Build history of the part. All positions in model axes, mm. Face numbers are marked on the shaded views. A direction names the side the tool comes from. Give positions to 0.01 mm unless a question says otherwise; leave off trailing zeros. Order: outer loops, then holes, each group sorted by start corner. A loop starts at its lowest first (then second) coordinate and runs counter-clockwise, first axis right, second up. Notation, with made-up numbers: (18.5, 55) -> (49.5, 55) arc R22 ccw to (49.5, 64) -> close; hole circle Ø11 at (11.5, -38.5). An arc over 180 degrees is marked (long way). One line per item, written item: value. Start each with the question number.
(1) Probe line 1 (Z direction, x = -115.5, y = -19.5); line 2 (Y direction, x = -63, z = 14); line 3 (Y direction, x = -143.5, z = 17.5). List the from-to ranges inside material, lowest first.
(2) Which spindle directions (+Z, -Z, +X, -X, +Y, -Y) get a long thin tool onto all of the face, cutting with end or side? Do the marked faces 1, 2 and 3. Say none if no direction does.
(3) Saw through at D-D on z = 23.5. Give the cut face in (x, y).
(4) Saw through at A-A on x = 24.5. Give the cut face in (y, z), plus the area to 3 significant figures.
(5) Pin check, flat tips, straight feed: pin 1 (1.5 mm diameter, centred on y = -13.5, z = 4, fed in from -X); pin 2 (4 mm diameter, centred on y = 19.5, z = 11, fed in from +X); pin 3 (8 mm diameter, centred on x = 22.5, z = 10, fed in from -Y). Stop position of each tip, or through.
(6) Two-plate mould, pull along Y, no slides. Class the marked faces 4, 5, 6 and 7: +Y half, -Y half, draft (parallel to the pull), parting line (faces both ways), or undercut.
(7) Saw through at C-C on x = -23. Give the cut face in (y, z), plus the area to 3 significant figures.
(8) Saw through at B-B on y = -61. Give the cut face in (x, z), plus the area to 3 significant figures.
```python
from build123d import *

# Parameters (mm, degrees)
BOSS_EXTRUDE1_DEPTH = 30
BOSS_EXTRUDE2_DEPTH = 2


with BuildPart() as part:
    # Sketch1 → Boss-Extrude1 (new body)
    with BuildSketch(Plane.XY):
        with BuildLine():
            ThreePointArc((-124.422839539, -52.93360637), (-124.888175134, -64.31939994), (-119.594822483, -74.410646153))
            Line((-119.594822483, -74.410646153), (-111.407238253, -83.286865316))
            Line((-111.407238253, -83.286865316), (35.730934718, -56.776536745))
            Line((35.730934718, -56.776536745), (37.30735825, -35.897821688))
            ThreePointArc((37.30735825, -35.897821688), (33.813482954, -35.461340503), (30.378958676, -34.685632184))
            Line((30.378958676, -34.685632184), (29.158639343, -50.847976334))
            Line((29.158639343, -50.847976334), (-108.867065108, -75.716483958))
            Line((-108.867065108, -75.716483958), (-114.449508902, -69.664516346))
            ThreePointArc((-114.449508902, -69.664516346), (-118.058612981, -62.784121201), (-117.741338712, -55.021080131))
            ThreePointArc((-117.741338712, -55.021080131), (-120.686835144, -35.887822689), (-137.611023, -26.489452883))
            ThreePointArc((-137.611023, -26.489452883), (-140.360427807, -25.849420576), (-142.716361529, -24.294285714))
            ThreePointArc((-142.716361529, -24.294285714), (-148.157403518, -8.953967174), (-139.001078611, 4.503076521))
            ThreePointArc((-139.001078611, 4.503076521), (-130.143335416, 13.552732011), (-127.741520279, 25.986040624))
            ThreePointArc((-127.741520279, 25.986040624), (-124.12688517, 37.354531527), (-113.359672518, 42.490220779))
            Line((-113.359672518, 42.490220779), (36.615125644, 47.908385572))
            Line((36.615125644, 47.908385572), (35.69634188, 35.73968597))
            ThreePointArc((35.69634188, 35.73968597), (39.20840278, 35.99090031), (42.728206295, 35.897821688))
            Line((42.728206295, 35.897821688), (44.184569482, 55.186414758))
            Line((44.184569482, 55.186414758), (-113.612397826, 49.485657143))
            ThreePointArc((-113.612397826, 49.485657143), (-129.404309715, 41.953312906), (-134.705774542, 25.279526249))
            ThreePointArc((-134.705774542, 25.279526249), (-136.343375771, 16.802270376), (-142.382746132, 10.632050724))
            ThreePointArc((-142.382746132, 10.632050724), (-155.099864059, -8.058287742), (-147.542861296, -29.364285714))
            ThreePointArc((-147.542861296, -29.364285714), (-143.125485566, -32.280163581), (-137.970351553, -33.480224156))
            ThreePointArc((-137.970351553, -33.480224156), (-126.431132561, -39.888203569), (-124.422839539, -52.93360637))
        make_face()
    extrude(amount=BOSS_EXTRUDE1_DEPTH)

    # Sketch4 → Boss-Extrude2 (add)
    with BuildSketch(Plane.XY.offset(30)):
        with BuildLine():
            Line((36.615125644, 47.908385572), (-113.359672518, 42.490220779))
            ThreePointArc((-113.359672518, 42.490220779), (-124.12688517, 37.354531527), (-127.741520279, 25.986040624))
            ThreePointArc((-127.741520279, 25.986040624), (-130.143335416, 13.552732011), (-139.001078611, 4.503076521))
            ThreePointArc((-139.001078611, 4.503076521), (-148.157403518, -8.953967174), (-142.716361529, -24.294285714))
            ThreePointArc((-142.716361529, -24.294285714), (-140.360427807, -25.849420576), (-137.611023, -26.489452883))
            ThreePointArc((-137.611023, -26.489452883), (-120.686835144, -35.887822689), (-117.741338712, -55.021080131))
            ThreePointArc((-117.741338712, -55.021080131), (-118.058612981, -62.784121201), (-114.449508902, -69.664516346))
            Line((-114.449508902, -69.664516346), (-108.867065108, -75.716483958))
            Line((-108.867065108, -75.716483958), (29.158639343, -50.847976334))
            Line((29.158639343, -50.847976334), (30.378958676, -34.685632184))
            ThreePointArc((30.378958676, -34.685632184), (4.119960585, 2.710424022), (35.69634188, 35.73968597))
            Line((35.69634188, 35.73968597), (36.615125644, 47.908385572))
        make_face()
        with BuildLine():
            ThreePointArc((-117.741338712, -55.021080131), (-120.686835144, -35.887822689), (-137.611023, -26.489452883))
            ThreePointArc((-137.611023, -26.489452883), (-140.360427807, -25.849420576), (-142.716361529, -24.294285714))
            ThreePointArc((-142.716361529, -24.294285714), (-148.157403518, -8.953967174), (-139.001078611, 4.503076521))
            ThreePointArc((-139.001078611, 4.503076521), (-130.143335416, 13.552732011), (-127.741520279, 25.986040624))
            ThreePointArc((-127.741520279, 25.986040624), (-124.12688517, 37.354531527), (-113.359672518, 42.490220779))
            Line((-113.359672518, 42.490220779), (36.615125644, 47.908385572))
            Line((36.615125644, 47.908385572), (35.69634188, 35.73968597))
            ThreePointArc((35.69634188, 35.73968597), (39.20840278, 35.99090031), (42.728206295, 35.897821688))
            Line((42.728206295, 35.897821688), (44.184569482, 55.186414758))
            Line((44.184569482, 55.186414758), (-113.612397826, 49.485657143))
            ThreePointArc((-113.612397826, 49.485657143), (-129.404309715, 41.953312906), (-134.705774542, 25.279526249))
            ThreePointArc((-134.705774542, 25.279526249), (-136.343375771, 16.802270376), (-142.382746132, 10.632050724))
            ThreePointArc((-142.382746132, 10.632050724), (-155.099864059, -8.058287742), (-147.542861296, -29.364285714))
            ThreePointArc((-147.542861296, -29.364285714), (-143.125485566, -32.280163581), (-137.970351553, -33.480224156))
            ThreePointArc((-137.970351553, -33.480224156), (-126.431132561, -39.888203569), (-124.422839539, -52.93360637))
            ThreePointArc((-124.422839539, -52.93360637), (-124.888175134, -64.31939994), (-119.594822483, -74.410646153))
            Line((-119.594822483, -74.410646153), (-111.407238253, -83.286865316))
            Line((-111.407238253, -83.286865316), (35.730934718, -56.776536745))
            Line((35.730934718, -56.776536745), (37.30735825, -35.897821688))
            ThreePointArc((37.30735825, -35.897821688), (33.813482954, -35.461340503), (30.378958676, -34.685632184))
            Line((30.378958676, -34.685632184), (29.158639343, -50.847976334))
            Line((29.158639343, -50.847976334), (-108.867065108, -75.716483958))
            Line((-108.867065108, -75.716483958), (-114.449508902, -69.664516346))
            ThreePointArc((-114.449508902, -69.664516346), (-118.058612981, -62.784121201), (-117.741338712, -55.021080131))
        make_face()
    extrude(amount=BOSS_EXTRUDE2_DEPTH)


solid = part.part
```
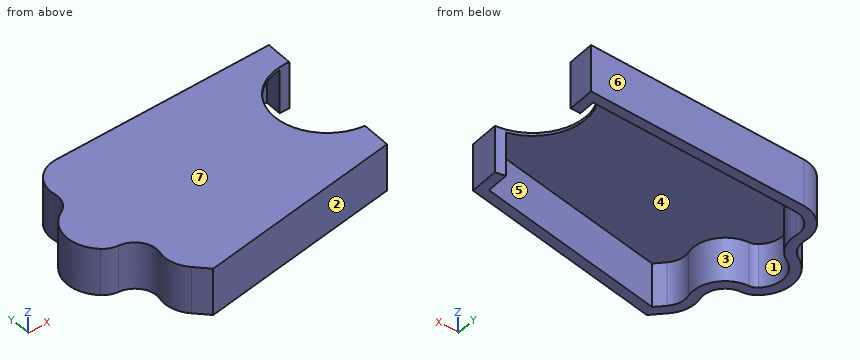
Results below:
1. line 1: z = 30 to 32
1. line 2: y = -74.57 to -67.45, 44.31 to 51.31
1. line 3: y = -32.11 to -23.5, 0.99 to 9.98
2. face 1: -Z, +X
2. face 2: +Z, -Z, +X, -Y
2. face 3: -Z
3. outline: (-147.54, -29.36) arc R15 ccw to (-137.97, -33.48) arc R15 cw to (-124.42, -52.93) arc R22 ccw to (-119.59, -74.41) -> (-111.41, -83.29) -> (35.73, -56.78) -> (37.31, -35.9) arc R36 cw to (30.38, -34.69) -> (29.16, -50.85) -> (-108.87, -75.72) -> (-114.45, -69.66) arc R15 cw to (-117.74, -55.02) arc R22 ccw to (-137.61, -26.49) arc R8 cw to (-142.72, -24.29) arc R18 cw to (-139, 4.5) arc R22 ccw to (-127.74, 25.99) arc R15 cw to (-113.36, 42.49) -> (36.62, 47.91) -> (35.7, 35.74) arc R36 cw to (42.73, 35.9) -> (44.18, 55.19) -> (-113.61, 49.49) arc R22 ccw to (-134.71, 25.28) arc R15 cw to (-142.38, 10.63) arc R25 ccw to start
4. outline: (-58.8, 0) -> (-51.69, 0) -> (-51.69, 30) -> (-32.48, 30) -> (-32.48, 32) -> (-58.8, 32) -> close; (32.48, 30) -> (47.47, 30) -> (47.47, 0) -> (54.48, 0) -> (54.48, 32) -> (32.48, 32) -> close
4. area: 520 mm²
5. pin 1: stops at x = -155.26
5. pin 2: stops at x = -127.75
5. pin 3: stops at y = -59.88
6. face 4: undercut
6. face 5: undercut
6. face 6: +Y half
6. face 7: draft
7. outline: (-67.36, 0) -> (-60.25, 0) -> (-60.25, 30) -> (45.75, 30) -> (45.75, 0) -> (52.76, 0) -> (52.76, 32) -> (-67.36, 32) -> close
7. area: 664 mm²
8. outline: (-125.37, 0) -> (-118.35, 0) -> (-118.35, 30) -> (-27.19, 30) -> (-27.19, 0) -> (12.29, 0) -> (12.29, 32) -> (-125.37, 32) -> close
8. area: 1,670 mm²
